Work out the finished part from the listing and answer in its coordinate system (mm). Face numbers are marked on the shaded views. A direction names the side the tool comes from. Round coordinates to 2 decimals unless told otherwise and drop trailing zeros. Loops run counter-clockwise (first coordinate to the right, second up) from the corner with the lowest first, then second, coordinate; pieces in that order, holes last.
```python
from build123d import *

# Parameters (mm, degrees)
F1_DEPTH = 50
F2_R     = 5


with BuildPart() as f1:
    # F0 (on Front) → F1 (new body, symmetric)
    with BuildSketch(Plane.XZ):
        with BuildLine():
            Line((19.05, 76.2), (-19.05, 76.2))
            ThreePointArc((-19.05, 76.2), (-23.5401280605, 74.3401280605), (-25.4, 69.85))
            Line((-25.4, 69.85), (-25.4, -69.85))
            ThreePointArc((-25.4, -69.85), (-23.5401280605, -74.3401280605), (-19.05, -76.2))
            ThreePointArc((-19.05, -76.2), (-14.5598719395, -74.3401280605), (-12.7, -69.85))
            Line((-12.7, -69.85), (-12.7, -63.5))
            Line((-12.7, -63.5), (-12.7, 57.15))
            ThreePointArc((-12.7, 57.15), (-10.8401280605, 61.6401280605), (-6.35, 63.5))
            Line((-6.35, 63.5), (6.35, 63.5))
            ThreePointArc((6.35, 63.5), (10.8401280605, 61.6401280605), (12.7, 57.15))
            Line((12.7, 57.15), (12.7, -63.5))
            Line((12.7, -63.5), (12.7, -69.85))
            ThreePointArc((12.7, -69.85), (14.5598719395, -74.3401280605), (19.05, -76.2))
            ThreePointArc((19.05, -76.2), (23.5401280605, -74.3401280605), (25.4, -69.85))
            Line((25.4, -69.85), (25.4, 69.85))
            ThreePointArc((25.4, 69.85), (23.5401280605, 74.3401280605), (19.05, 76.2))
        make_face()
    extrude(amount=F1_DEPTH, both=True)

    # F2
    f2_edges = [f1.edges().sort_by_distance(p)[0] for p in [
        (19.05, 50, -76.2),
        (25.4, 50, 0),
        (23.540128, 50, 74.340128),
        (0, 50, 76.2),
        (-23.540128, 50, 74.340128),
        (-25.4, 50, 0),
        (-19.05, 50, -76.2),
        (-12.7, 50, -6.35),
        (-10.840128, 50, 61.640128),
        (0, 50, 63.5),
        (10.840128, 50, 61.640128),
        (12.7, 50, -6.35),
        (19.05, -50, -76.2),
    ]]
    fillet(f2_edges, radius=F2_R)


solid = f1.part
```
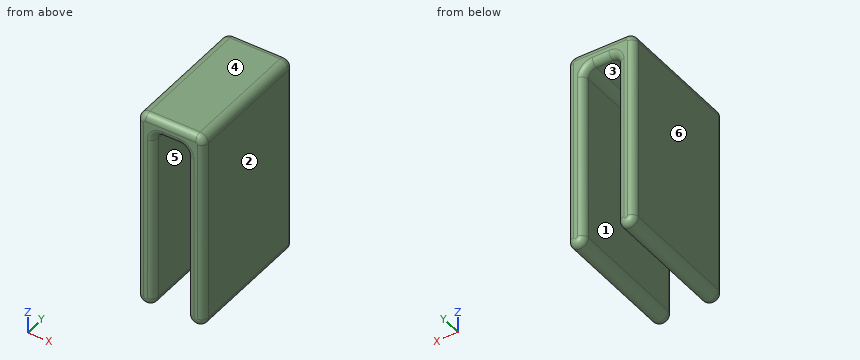
1. Which of the six approach directions +Z, -Z, +X, -X, +Y, -Y give full straight-line access (tool end or side, diameter ignored) to the marked faces 1 and 2?
Answer key:
face 1: -Z, +Y, -Y
face 2: +Z, -Z, +X, +Y, -Y
2. Consider probe 1 along X at (y, z) = (17, 47); probe 2 along Z at (x, y) = (-5.5, 22.5); probe 3 along X at (y, z) = (46, -3). Determine where each line is inside the solid, lowest interval first.
Answer key:
probe 1: x = -25.4 to -12.7, 12.7 to 25.4
probe 2: z = 63.5 to 76.2
probe 3: x = -25.3 to -12.8, 12.8 to 25.3
3. Find section B-B (y = -22). Write down the section's boundary in (x, z), then the cut area to 3 significant figures.
Answer key:
outline: (-25.4, -69.85) arc R6.35 ccw to (-12.7, -69.85) - (-12.7, 57.15) arc R6.35 cw to (-6.35, 63.5) - (6.35, 63.5) arc R6.35 cw to (12.7, 57.15) - (12.7, -69.85) arc R6.35 ccw to (25.4, -69.85) - (25.4, 69.85) arc R6.35 ccw to (19.05, 76.2) - (-19.05, 76.2) arc R6.35 ccw to (-25.4, 69.85) - close
area: 4,160 mm2
4. Find section C-C (x = 2). Write down the section's boundary in (y, z).
Answer key:
outline: (-50, 68.5) arc R5 ccw to (-45, 63.5) - (45, 63.5) arc R5 ccw to (50, 68.5) - (50, 71.2) arc R5 ccw to (45, 76.2) - (-45, 76.2) arc R5 ccw to (-50, 71.2) - close
5. Find section A-A (z = -20). Write down the section's boundary in (x, y).
Answer key:
outline: (-25.4, -45) arc R5 ccw to (-20.4, -50) - (-17.7, -50) arc R5 ccw to (-12.7, -45) - (-12.7, 45) arc R5 ccw to (-17.7, 50) - (-20.4, 50) arc R5 ccw to (-25.4, 45) - close; (12.7, -45) arc R5 ccw to (17.7, -50) - (20.4, -50) arc R5 ccw to (25.4, -45) - (25.4, 45) arc R5 ccw to (20.4, 50) - (17.7, 50) arc R5 ccw to (12.7, 45) - close
6. Given pin 1 (14 mm diameter, centred on x = -1.5, y = -4, fed in from -Z); pin 2 (1.5 mm diameter, centred on x = 1.5, y = -10, fed in from -Z), each flat-ended and moving along its own axis, determine where each tip first touches the part or whether it passes through.
Answer key:
pin 1: stops at z = 63.12
pin 2: stops at z = 63.5
7. Determine the mould class of the marked faces 3, 4, 5 and 6 for opening direction X: +X half, -X half, draft (parallel to the pull), parting line (faces both ways), or undercut.
Answer key:
face 3: undercut
face 4: draft
face 5: undercut
face 6: -X half
